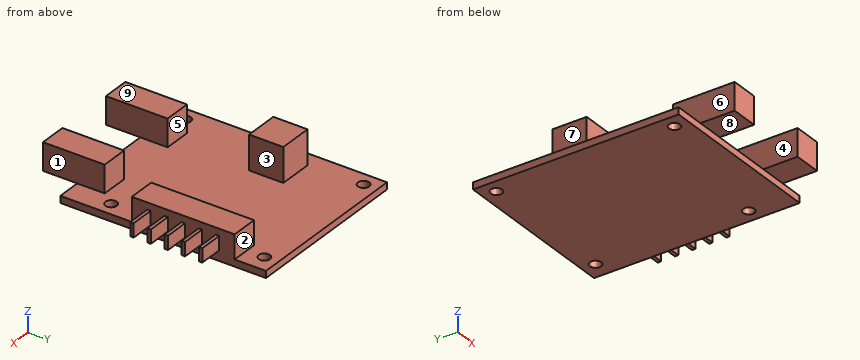
from build123d import *

# Parameters (mm, degrees)
ESQUISSE1_W        = 50
ESQUISSE1_H        = 60
ESQUISSE1_R        = 1.65
BOSS_EXTRU_1_DEPTH = 2
ESQUISSE2_W        = 8
ESQUISSE2_H        = 18
BOSS_EXTRU_2_DEPTH = 8
ESQUISSE3_W        = 10
ESQUISSE3_H        = 10
BOSS_EXTRU_3_DEPTH = 10
ESQUISSE4_W        = 8
ESQUISSE4_H        = 30
BOSS_EXTRU_4_DEPTH = 7
ESQUISSE5_W        = 4
ESQUISSE5_H        = 1
BOSS_EXTRU_5_DEPTH = 7


with BuildPart() as part:
    # Esquisse1 → Boss.-Extru.1 (new body)
    with BuildSketch(Plane.XY):
        with Locations((1.490133333, 29.802666667)):
            Rectangle(ESQUISSE1_W, ESQUISSE1_H)
        with Locations((-19.509866667, 55.802666667)):
            Circle(ESQUISSE1_R, mode=Mode.SUBTRACT)
        with Locations((21.490133333, 55.802666667)):
            Circle(ESQUISSE1_R, mode=Mode.SUBTRACT)
        with Locations((22.490133333, 11.802666667)):
            Circle(ESQUISSE1_R, mode=Mode.SUBTRACT)
        with Locations((-19.509866667, 3.802666667)):
            Circle(ESQUISSE1_R, mode=Mode.SUBTRACT)
    extrude(amount=BOSS_EXTRU_1_DEPTH)

    # Esquisse2 → Boss.-Extru.2 (add)
    with BuildSketch(Plane.XY.offset(2)):
        with Locations((-10.509866667, -1.197333333)):
            Rectangle(ESQUISSE2_W, ESQUISSE2_H)
        with Locations((15.490133333, -1.197333333)):
            Rectangle(ESQUISSE2_W, ESQUISSE2_H)
    extrude(amount=BOSS_EXTRU_2_DEPTH)

    # Esquisse3 → Boss.-Extru.3 (add)
    with BuildSketch(Plane.XY.offset(2)):
        with Locations((-14.009866667, 34.802666667)):
            Rectangle(ESQUISSE3_W, ESQUISSE3_H)
    extrude(amount=BOSS_EXTRU_3_DEPTH)

    # Esquisse4 → Boss.-Extru.4 (add)
    with BuildSketch(Plane.XY.offset(2)):
        with Locations((22.490133333, 35.662666667)):
            Rectangle(ESQUISSE4_W, ESQUISSE4_H)
    extrude(amount=BOSS_EXTRU_4_DEPTH)

    # Esquisse5 → Boss.-Extru.5 (add)
    with BuildSketch(Plane(origin=(26.490133333, 0, 0), x_dir=(0, 0, -1), z_dir=(1, 0, 0))):
        with Locations((-5, 35.662666667)):
            Rectangle(ESQUISSE5_W, ESQUISSE5_H)
        with Locations((-5, 40.662666667)):
            Rectangle(ESQUISSE5_W, ESQUISSE5_H)
        with Locations((-5, 45.662666667)):
            Rectangle(ESQUISSE5_W, ESQUISSE5_H)
        with Locations((-5, 30.662666667)):
            Rectangle(ESQUISSE5_W, ESQUISSE5_H)
        with Locations((-5, 25.662666667)):
            Rectangle(ESQUISSE5_W, ESQUISSE5_H)
    extrude(amount=BOSS_EXTRU_5_DEPTH)


solid = part.part
CAD build for the part. Positions are in the model's coordinates, mm. Face numbers are marked on the shaded views. A direction names the side the tool comes from. Coordinates: 2 decimals unless noted, no trailing zeros. Loops run counter-clockwise (first coordinate to the right, second up) from the corner with the lowest first, then second, coordinate; pieces in that order, holes last. Notation, with made-up numbers: (41.25, -8.75) -> (48.25, -8.75) arc R22 ccw to (48.25, 24.25) -> close; hole circle Ø7 at (8.5, -1.75). An arc over 180 degrees is marked (long way). One line per item, written item: value.
1. Slice it at A-A on y = -5. Write the cut outline in (x, z).
Answers:
outline: (-14.51, 2) -> (-6.51, 2) -> (-6.51, 10) -> (-14.51, 10) -> close; (11.49, 2) -> (19.49, 2) -> (19.49, 10) -> (11.49, 10) -> close
2. Slice it at C-C on y = 24. Write the cut outline in (x, z), and give its area (3 significant figures).
Answers:
outline: (-23.51, 0) -> (26.49, 0) -> (26.49, 9) -> (18.49, 9) -> (18.49, 2) -> (-23.51, 2) -> close
area: 156 mm^2
3. Drill centre lines: line 1 (X direction, y = 36, z = 6); line 2 (X direction, y = 32.5, z = 2.25); line 3 (Z direction, x = 9, y = 30.5). Where is each one in solid material? Low to high. Write a range as [from, to].
Answers:
line 1: x = [-19.01, -9.01], [18.49, 33.49]
line 2: x = [-19.01, -9.01], [18.49, 26.49]
line 3: z = [0, 2]
4. Slice it at B-B on x = -16. Write the cut outline in (y, z), and give its area (3 significant figures).
Answers:
outline: (-0.2, 0) -> (59.8, 0) -> (59.8, 2) -> (39.8, 2) -> (39.8, 12) -> (29.8, 12) -> (29.8, 2) -> (-0.2, 2) -> close
area: 220 mm^2
5. Pull direction X, two halves, no side cores. Call the marked faces 1, 2, 3 and 4: pulls with the +X half, pulls with the -X half, needs draft (parallel to the pull), parting line crosses it, or undercut.
Answers:
face 1: pulls with the +X half
face 2: needs draft
face 3: undercut
face 4: undercut
6. Slice it at D-D on z = 10.75. Write the cut outline in (x, y).
Answers:
outline: (-19.01, 29.8) -> (-9.01, 29.8) -> (-9.01, 39.8) -> (-19.01, 39.8) -> close
7. Flat gauge pins, fed straight in: P1, Ø0.5, axis at x = 31, y = 30.5, coming from the -Z side; P2, Ø5, axis at x = -16, z = 6, coming from the +Y side; P3, Ø4.5, axis at x = -19.51, y = 3.8, coming from the +Z side. Where does each tip first touch, or does it go through?
Answers:
P1: stops at z = 3
P2: stops at y = 39.8
P3: stops at z = 2
8. Which spindle directions (+Z, -Z, +X, -X, +Y, -Y) get a long thin tool onto all of the face, cutting with end or side? Do the marked faces 5, 6, 7, 8 and 9. Say none if no direction does.
Answers:
face 5: +Z, +X, -X
face 6: +Z, -X, -Y
face 7: +Z, -X, +Y, -Y
face 8: -Z, +X, -X, -Y
face 9: +Z, +X, -X, -Y
